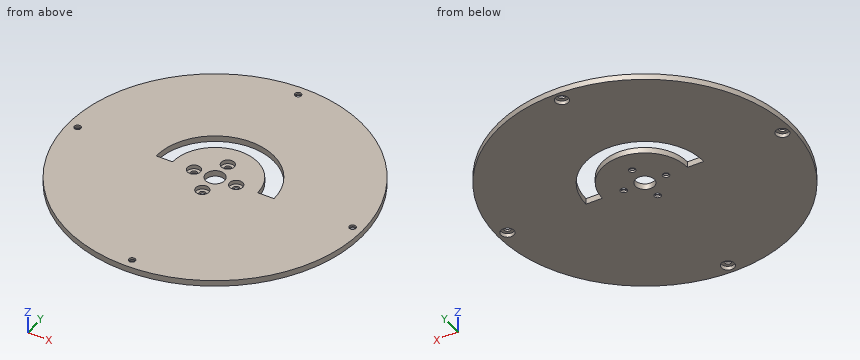
```python
from build123d import *

# Parameters (mm, degrees)
SKETCH_R        = 45
SKETCH_R_2      = 1
SKETCH_R_3      = 2.9
PAD_DEPTH       = 1.8
SKETCH001_R     = 2
POCKET_DEPTH    = 1.2
SKETCH002_R     = 1
POCKET001_DEPTH = 1.801
SKETCH003_R     = 2
POCKET002_DEPTH = 1.2
POCKET003_DEPTH = 1.801


with BuildPart() as part:
    # Sketch → Pad (new body)
    with BuildSketch(Plane.XY):
        Circle(SKETCH_R)
        with Locations((0, 6.45)):
            Circle(SKETCH_R_2, mode=Mode.SUBTRACT)
        with Locations((-6.45, 0)):
            Circle(SKETCH_R_2, mode=Mode.SUBTRACT)
        with Locations((6.45, 0)):
            Circle(SKETCH_R_2, mode=Mode.SUBTRACT)
        with Locations((0, -6.45)):
            Circle(SKETCH_R_2, mode=Mode.SUBTRACT)
        Circle(SKETCH_R_3, mode=Mode.SUBTRACT)
    extrude(amount=PAD_DEPTH)

    # Sketch001 → Pocket (cut)
    with BuildSketch(Plane.XY.offset(1.8)):
        with Locations((-6.45, 0)):
            Circle(SKETCH001_R)
        with Locations((0, 6.45)):
            Circle(SKETCH001_R)
        with Locations((6.45, 0)):
            Circle(SKETCH001_R)
        with Locations((0, -6.45)):
            Circle(SKETCH001_R)
    extrude(amount=-POCKET_DEPTH, mode=Mode.SUBTRACT)

    # Sketch002 → Pocket001 (cut, through all)
    with BuildSketch(Plane.XY.offset(1.8)):
        with Locations((-42, 0)):
            Circle(SKETCH002_R)
        with Locations((42, 0)):
            Circle(SKETCH002_R)
        with Locations((0, 42)):
            Circle(SKETCH002_R)
        with Locations((0, -42)):
            Circle(SKETCH002_R)
    extrude(amount=-POCKET001_DEPTH, mode=Mode.SUBTRACT)

    # Sketch003 → Pocket002 (cut)
    with BuildSketch(Plane(origin=(0, 0, 0), x_dir=(1, 0, 0), z_dir=(0, 0, -1))):
        with Locations((-42, 0)):
            Circle(SKETCH003_R)
        with Locations((0, 42)):
            Circle(SKETCH003_R)
        with Locations((42, 0)):
            Circle(SKETCH003_R)
        with Locations((0, -42)):
            Circle(SKETCH003_R)
    extrude(amount=-POCKET002_DEPTH, mode=Mode.SUBTRACT)

    # Sketch004 → Pocket003 (cut, through all)
    with BuildSketch(Plane(origin=(0, 0, 0), x_dir=(1, 0, 0), z_dir=(0, 0, -1))):
        with BuildLine():
            ThreePointArc((-13, 0), (0, -13), (13, 0))
            Line((13, 0), (18, 0))
            ThreePointArc((-18, 0), (0, -18), (18, 0))
            Line((-18, 0), (-13, 0))
        make_face()
    extrude(amount=-POCKET003_DEPTH, mode=Mode.SUBTRACT)


solid = part.part
```
Model file for the job. Use its own axes, mm. Give positions to 0.01 mm unless a question says otherwise; leave off trailing zeros. Loops run counter-clockwise (first coordinate to the right, second up) from the corner with the lowest first, then second, coordinate; pieces in that order, holes last. Notation, with made-up numbers: (57.5, 89) -> (98.5, 89) arc R9 cw to (98.5, 105) -> close; hole circle Ø3 at (44, 35.5). An arc over 180 degrees is marked (long way). Use CSV: the item, a comma, the result in double quotes. Start each with the question number.
1) Wall check: line 1 (Y direction, x = -6, z = 1.6); line 2 (X direction, y = -0.5, z = 1.5); line 3 (X direction, y = 7.5, z = 0.8). Give the ranges that are in metal, low to high.
2) Slice it at A-A on x = 29. Give the cut face in (y, z).
3) Slice it at B-B on y = -38. Give the cut face in (x, z), plus the area to 3 significant figures.
4) Flat gauge pins, fed straight in: pin 1 Ø0.9 at (x, z) = (-14.5, 1) entering from +Y; pin 2 Ø1.6 at (x, y) = (-42, 0) entering from -Z; pin 3 Ø3.5 at (x, y) = (0, -6.45) entering from +Z. Where does each tip first touch, or does it go through?
Computed values:
1,line 1,"y = -44.6 to -1.95, 1.95 to 11.53, 16.97 to 44.6"
1,line 2,"x = -45 to -42.87, -41.13 to -8.39, -4.51 to -2.86, 2.86 to 4.51, 8.39 to 41.13, 42.87 to 45"
1,line 3,"x = -44.37 to -16.36, -10.62 to -1.7, 1.7 to 10.62, 16.36 to 44.37"
2,outline,"(-34.41, 0) -> (34.41, 0) -> (34.41, 1.8) -> (-34.41, 1.8) -> close"
3,outline,"(-24.1, 0) -> (24.1, 0) -> (24.1, 1.8) -> (-24.1, 1.8) -> close"
3,area,"86.8 mm^2"
4,pin 1,"stops at y = 42.75"
4,pin 2,"passes through"
4,pin 3,"stops at z = 0.6"
